Part model, mm, in its own coordinate system. A direction names the side the tool comes from. Give positions to 0.01 mm unless a question says otherwise; leave off trailing zeros. Order: outer loops, then holes, each group sorted by start corner. A loop starts at its lowest first (then second) coordinate and runs counter-clockwise, first axis right, second up. Notation, with made-up numbers: M 61.25,39.5 L 118.25,39.5 A24 cw 118.25,52.5 Z; hole C -12,-31.5 d6. An arc over 180 degrees is marked long. Write each question's results on one line, items separated by ' | '. Start each with the question number.
from build123d import *

# Parameters (mm, degrees)
CHANFREIN1_SIZE = 1
PER_AGE1_D      = 3
PER_AGE1_DEPTH  = 25
PER_AGE1_TIP    = 0.901290929


with BuildPart() as part:
    # Esquisse1 → Base-Révolution (revolve)
    with BuildSketch(Plane.XY, mode=Mode.PRIVATE) as base_r_volution_sk:
        with BuildLine():
            Line((0, 0), (0, -9))
            Line((0, -9), (2, -9))
            Line((2, -9), (2, -7.75))
            Line((2, -7.75), (23.085786438, -7.75))
            ThreePointArc((23.085786438, -7.75), (24.5, -7.25), (25.914213562, -7.75))
            Line((25.914213562, -7.75), (107, -7.75))
            Line((107, -7.75), (109.5, -6.75))
            Line((109.5, -6.75), (109.5, -4.5))
            Line((109.5, -4.5), (118, -4.5))
            Line((118, -4.5), (118, 0))
            Line((118, 0), (0, 0))
        make_face()
    revolve(base_r_volution_sk.sketch.rotate(Axis((-10, 0, 0), (1, 0, 0)), 270), axis=Axis((-10, 0, 0), (1, 0, 0)))

    # Chanfrein1
    chanfrein1_edges = [part.edges().sort_by_distance(p)[0] for p in [
        (0, 0, -9),
        (118, 0, -4.5),
    ]]
    chamfer(chanfrein1_edges, length=CHANFREIN1_SIZE)

    # Perçage1
    with Locations(Plane(origin=(118, 0, 0), x_dir=(0, 0, -1), z_dir=(1, 0, 0))):
        with Locations((0, 0)):
            Hole(PER_AGE1_D / 2, depth=PER_AGE1_DEPTH)
            with Locations((0, 0, -(PER_AGE1_DEPTH + PER_AGE1_TIP / 2))):  # 118° drill point
                Cone(0, PER_AGE1_D / 2, PER_AGE1_TIP, mode=Mode.SUBTRACT)


solid = part.part
(1) Probe L1, parallel to Y at x = 111.25, z = 0; L2, parallel to Y at x = 98.5, z = 0; L3, parallel to X at y = 5.25, z = 4.25. List the from-to ranges inside material, lowest first.
(2) Saw through at A-A on x = 83.5. Give the cut face in (y, z), plus the area to 3 significant figures.
(3) Tool access for faces 1 (the flat face through (0, 0, 0)), 2 (the cylindrical face through (113.302, -1.352, 4.292)): list every direction of +Z, -Z, +X, -X, +Y, -Y with a clear straight run to the whole face (end or side of a thin tool).
(4) Drop flat-ended pins along their axis: P1, Ø4, axis at x = 105.5, y = -4.5, coming from the -Z side; P2, Ø3, axis at x = 96, y = 6, coming from the +Z side; P3, Ø3, axis at y = 3, z = -5, coming from the +X side. Give the stop position or say it passes through.
(5) Pull direction Z, two halves, no side cores. Call faces 3 (the cylindrical face through (67.025, -7.684, -1.009)), 4 (the flat face through (109.5, 4.4, -1.6)), 5 (the cylindrical face through (105.32, 0.07, -1.5)): +Z half, -Z half, draft (parallel to the pull), parting line (faces both ways), or undercut.
Taken from the geometry:
1) L1: y = -4.5 to -1.5, 1.5 to 4.5 | L2: y = -7.75 to -1.5, 1.5 to 7.75 | L3: x = 0 to 109.49
2) outline: C 0,0 d15.5 | area: 189 mm²
3) face 1: +Z, -Z, -X, +Y, -Y | face 2: +X
4) P1: stops at z = -7.34 | P2: stops at z = 6.31 | P3: stops at x = 117.17
5) face 3: parting line | face 4: draft | face 5: undercut
